```python
from build123d import *

# Parameters (mm, degrees)
SALIENTE_EXTRUIR1_START = 80
SALIENTE_EXTRUIR1_DEPTH = 3
SALIENTE_EXTRUIR2_START = 40
SALIENTE_EXTRUIR2_DEPTH = 40
SALIENTE_EXTRUIR3_START = -80
CROQUIS3_W              = 80
CROQUIS3_H              = 128.485281374
SALIENTE_EXTRUIR3_DEPTH = 3
SALIENTE_EXTRUIR4_DEPTH = 40
SALIENTE_EXTRUIR5_START = 84.5
CROQUIS5_W              = 163
CROQUIS5_H              = 80
SALIENTE_EXTRUIR5_DEPTH = 4
SALIENTE_EXTRUIR6_START = -3
SALIENTE_EXTRUIR6_DEPTH = 3
SALIENTE_EXTRUIR7_START = 88.5
CROQUIS7_W              = 15
CROQUIS7_H              = 50
SALIENTE_EXTRUIR7_DEPTH = 50
CROQUIS8_R              = 9
SALIENTE_EXTRUIR8_DEPTH = 157
CROQUIS10_R             = 3
CORTAR_EXTRUIR1_DEPTH   = 20
CORTAR_EXTRUIR2_START   = -20
CROQUIS11_R             = 3
CORTAR_EXTRUIR2_DEPTH   = 20


with BuildPart() as part:
    # Croquis1 → Saliente-Extruir1 (new body)
    with BuildSketch(Plane(origin=(0, 0, 0), x_dir=(0, 0, -1), z_dir=(1, 0, 0)).offset(SALIENTE_EXTRUIR1_START)):
        Polygon((-40, 8.485281374), (-40, -40), (40, -40), (40, 8.485281374), (40, 40), (40, 88.485281374), (-40, 88.485281374), (-40, 40), align=None)
        with BuildLine():
            Line((-3, 12), (0, 12))
            Line((0, 12), (3, 12))
            Line((3, 12), (3, 8.485281374))
            ThreePointArc((3, 8.485281374), (0, -9), (-3, 8.485281374))
            Line((-3, 8.485281374), (-3, 12))
        make_face(mode=Mode.SUBTRACT)
    extrude(amount=SALIENTE_EXTRUIR1_DEPTH)

    # Croquis2 → Saliente-Extruir2 (add)
    with BuildSketch(Plane.ZY.offset(-80).offset(SALIENTE_EXTRUIR2_START)):
        with BuildLine():
            Line((3, 8.485281374), (3, 10.583005244))
            ThreePointArc((3, 10.583005244), (0, -11), (-3, 10.583005244))
            Line((-3, 10.583005244), (-3, 8.485281374))
            ThreePointArc((-3, 8.485281374), (0, -9), (3, 8.485281374))
        make_face()
    extrude(amount=-SALIENTE_EXTRUIR2_DEPTH)



with BuildPart() as body_2:
    # Croquis3 → Saliente-Extruir3 (new body)
    with BuildSketch(Plane(origin=(0, 0, 0), x_dir=(0, 0, -1), z_dir=(1, 0, 0)).offset(SALIENTE_EXTRUIR3_START)):
        with Locations((0, 24.242640687)):
            Rectangle(CROQUIS3_W, CROQUIS3_H)
    extrude(amount=SALIENTE_EXTRUIR3_DEPTH)

    # Croquis4 → Saliente-Extruir4 (add)
    with BuildSketch(Plane(origin=(-77, 0, 0), x_dir=(0, 0, -1), z_dir=(1, 0, 0))):
        with BuildLine():
            Line((-3, 10.583005244), (-3, 8.485281374))
            ThreePointArc((-3, 8.485281374), (0, -9), (3, 8.485281374))
            Line((3, 8.485281374), (3, 10.583005244))
            ThreePointArc((3, 10.583005244), (0, -11), (-3, 10.583005244))
        make_face()
    extrude(amount=SALIENTE_EXTRUIR4_DEPTH)


with BuildPart() as part_1:
    add(part.part)

    add(body_2.part)  # Saliente-Extruir5 merges body 2
    # Croquis5 → Saliente-Extruir5 (add)
    with BuildSketch(Plane(origin=(0, 0, 0), x_dir=(1, 0, 0), z_dir=(0, 1, 0)).offset(SALIENTE_EXTRUIR5_START)):
        with Locations((1.5, 0)):
            Rectangle(CROQUIS5_W, CROQUIS5_H)
    extrude(amount=SALIENTE_EXTRUIR5_DEPTH)

    # Croquis6 → Saliente-Extruir6 (add)
    with BuildSketch(Plane(origin=(83, 0, 0), x_dir=(0, 0, -1), z_dir=(1, 0, 0)).offset(SALIENTE_EXTRUIR6_START)):
        with BuildLine():
            Line((3, 12), (3, 8.485281374))
            ThreePointArc((3, 8.485281374), (0, -9), (-3, 8.485281374))
            Line((-3, 8.485281374), (-3, 12))
            Line((-3, 12), (3, 12))
        make_face()
    extrude(amount=SALIENTE_EXTRUIR6_DEPTH)

    # Croquis7 → Saliente-Extruir7 (add)
    with BuildSketch(Plane(origin=(0, 0, 0), x_dir=(1, 0, 0), z_dir=(0, 1, 0)).offset(SALIENTE_EXTRUIR7_START)):
        with Locations((-87.5, 0)):
            Rectangle(CROQUIS7_W, CROQUIS7_H)
        with Locations((90.5, 0)):
            Rectangle(CROQUIS7_W, CROQUIS7_H)
    extrude(amount=-SALIENTE_EXTRUIR7_DEPTH)

    # Croquis8 → Saliente-Extruir8 (add)
    with BuildSketch(Plane(origin=(-77, 0, 0), x_dir=(0, 0, -1), z_dir=(1, 0, 0))):
        with Locations(Location((0, 0, 0), (0, 0, 109.471220634))):
            Circle(CROQUIS8_R)
    extrude(amount=SALIENTE_EXTRUIR8_DEPTH)

    # Croquis10 → Cortar-Extruir1 (cut)
    with BuildSketch(Plane.ZY.offset(80)):
        Circle(CROQUIS10_R)
    extrude(amount=-CORTAR_EXTRUIR1_DEPTH, mode=Mode.SUBTRACT)

    # Croquis11 → Cortar-Extruir2 (cut)
    with BuildSketch(Plane(origin=(83, 0, 0), x_dir=(0, 0, -1), z_dir=(1, 0, 0)).offset(CORTAR_EXTRUIR2_START)):
        with Locations(Location((0, 0, 0), (0, 0, 180))):
            Circle(CROQUIS11_R)
    extrude(amount=CORTAR_EXTRUIR2_DEPTH, mode=Mode.SUBTRACT)


solid = part_1.part
```
The listing builds one solid part. Answer for the finished solid, in the listing's coordinates (mm). A direction names the side the tool comes from. Round coordinates to 2 decimals unless told otherwise and drop trailing zeros. Write each loop counter-clockwise with the first axis right and the second up, starting at its lowest first coordinate (ties: lowest second). Pieces come first, ordered by that corner, then holes. Notation, with made-up numbers: (30, 54.25) -> (89, 54.25) arc R18 cw to (89, 67.25) -> close; hole circle Ø1 at (-31.5, -12.5). An arc over 180 degrees is marked (long way). Use CSV: the item, a comma, the result in double quotes. Start each with the question number.
(1) Section C-C on x = -41.5 is taken. Give the vertices of the cut face in (y, z), then the cut area to 3 significant figures.
(2) The mould has two halves that part along X. Classify faces 5 (the face through (60, -11, 0)), 6 (the face through (72.86, -0.9, 2.86)), 7 (the face through (98, 64, 0)): released by +X, released by -X, zero draft, split by the parting line, or undercut.
(3) Consider L1, parallel to Y at x = 68, z = 0; L2, parallel to X at y = -19.5, z = 6.5; L3, parallel to X at y = 44.5, z = -6. Determine where each line is inside the solid, lowest interval first. Write a range as from..to.
(4) Section B-B on y = 55 is taken. Give the vertices of the cut face in (x, z).
(5) Which of the six approach directions +Z, -Z, +X, -X, +Y, -Y give full straight-line access (tool end or side, diameter ignored) to faces 1 (the face through (-57, -11, 0)), 2 (the face through (-88, 38.5, 0)), 3 (the face through (90, 38.5, 0)), 4 (the face through (-70, 0, -3))?
(6) Each of these flat-tipped pins is pushed along its axis until it touches: pin 1 (3.5 mm diameter, centred on y = 0, z = 0, fed in from -X); pin 2 (8 mm diameter, centred on y = 0, z = 0, fed in from +X); pin 3 (12 mm diameter, centred on x = 93.5, y = 69.5, fed in from -Z); pin 4 (12 mm diameter, centred on x = -67, y = 18, fed in from -Z). Where does it stop, or does it pass through?
(7) Section A-A on z = 0 is taken. Give the vertices of the cut face in (x, y).
(8) Section D-D on z = 29.5 is taken. Give the vertices of the cut face in (x, y).
A:
1,outline,"(8.49, -3) arc R9 ccw to (8.49, 3) -> (10.58, 3) arc R11 ccw (long way) to (10.58, -3) -> close; (84.5, -40) -> (88.5, -40) -> (88.5, 40) -> (84.5, 40) -> close"
1,area,"688 mm²"
2,face 5,"undercut"
2,face 6,"zero draft"
2,face 7,"released by +X"
3,L1,"y = -11..-3, 3..9, 84.5..88.5"
3,L2,"x = -80..-77, 80..83"
3,L3,"x = -95..-77, 80..98"
4,outline,"(-95, -25) -> (-80, -25) -> (-80, -40) -> (-77, -40) -> (-77, 40) -> (-80, 40) -> (-80, 25) -> (-95, 25) -> close; (80, -40) -> (83, -40) -> (83, -25) -> (98, -25) -> (98, 25) -> (83, 25) -> (83, 40) -> (80, 40) -> close"
5,face 1,"none"
5,face 2,"+Z, -Z, -X, -Y"
5,face 3,"+Z, -Z, +X, -Y"
5,face 4,"-X"
6,pin 1,"stops at x = -60"
6,pin 2,"stops at x = 83"
6,pin 3,"stops at z = -25"
6,pin 4,"passes through"
7,outline,"(-95, 38.5) -> (-80, 38.5) -> (-80, 3) -> (-60, 3) -> (-60, -3) -> (-80, -3) -> (-80, -40) -> (-77, -40) -> (-77, -11) -> (-37, -11) -> (-37, -9) -> (40, -9) -> (40, -11) -> (80, -11) -> (80, -40) -> (83, -40) -> (83, -3) -> (63, -3) -> (63, 3) -> (83, 3) -> (83, 38.5) -> (98, 38.5) -> (98, 88.5) -> (-95, 88.5) -> close; hole (-77, 9) -> (80, 9) -> (80, 84.5) -> (-77, 84.5) -> close"
8,outline,"(-80, -40) -> (-77, -40) -> (-77, 84.5) -> (80, 84.5) -> (80, -40) -> (83, -40) -> (83, 88.5) -> (-80, 88.5) -> close"
